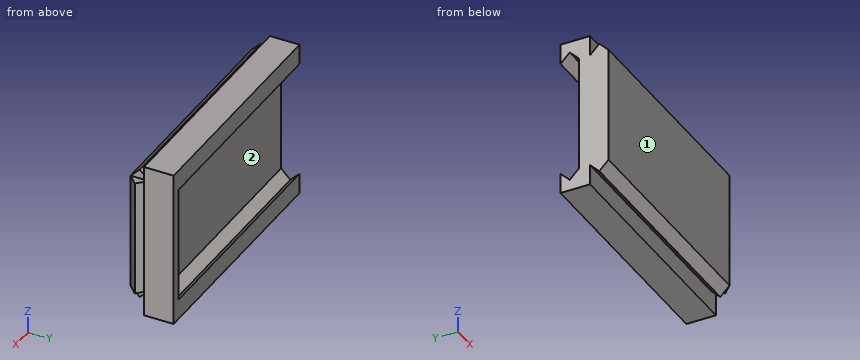
Autodesk Inventor part; units mm, degrees
ref_plane "Work Plane2" through (0, 0, 15.75) normal (0, 0, 1) x (1, 0, 0)
ref_plane "YZ Plane" through (0, 0, 0) normal (1, 0, 0) x (0, 1, 0)
ref_plane "XZ Plane" through (0, 0, 0) normal (0, 1, 0) x (-1, 0, 0)
sketch "Sketch5" plane through (0, 0, 0) normal (0, 0, 1) x (1, 0, 0)
  line L0 (-32, -5) -> (32, -5)
  line L1 (32, -5) -> (32, 5)
  line L2 (32, 5) -> (-32, 5)
  line L3 (-32, 5) -> (-32, -5)
  line L4 (-32, -5) -> (32, 5) construction
  line L5 (32, -5) -> (-32, 5) construction
  point P0 (0, 0)
  dimension "d17" = 64
  dimension "d18" = 10
extrude "Extrusion5" add sketch "Sketch5" along normal mid plane 46.5
ref_plane "Work Plane2" through (0, 0, 15.75) normal (0, 0, 1) x (1, 0, 0)
sketch "Sketch7" plane through (0, 0, 15.75) normal (0, 0, 1) x (1, 0, 0)
  line L0 (32, 5) -> (-32, 5)
  line L1 (-32, 5) -> (-32, -5)
  line L2 (-32, -5) -> (32, -5)
  line L3 (32, -5) -> (32, 5)
  line L4 (32, -5) -> (32, 5)
  line L5 (-32, -5) -> (32, -5)
  line L6 (32, 5) -> (-32, 5)
  line L7 (29.5, 5) -> (29.5, 0)
  line L8 (29.5, 5) -> (32, 2.5)
  line L9 (32, 2.5) -> (29.5, 0)
  point P0 (0, 0)
extrude "Extrusion6" cut sketch "Sketch7" against normal blind 31.5 contours L8 L9 L7
sketch "Sketch8" plane through (-32, -5, 23.25) normal (-1, 0, 0) x (0, 0, 1)
  line L0 (-46.5, 10) -> (0, 10)
  line L1 (-46.5, 10) -> (-41.5, 10)
  line L2 (-41.5, 0) -> (-46.5, 0)
  line L3 (-46.5, 5) -> (-46.5, 10)
  line L4 (0, 10) -> (-5, 10)
  line L5 (-46.5, 0) -> (-46.5, 10)
  line L6 (-41.5, 10) -> (-39, 10)
  line L7 (-39, 10) -> (-41.5, 7.5)
  line L8 (-39, 7.5) -> (-39, 5)
  line L9 (-39, 5) -> (-41.5, 7.5)
  line L10 (-5, 10) -> (-7.5, 10)
  line L11 (-7.5, 10) -> (-5, 7.5)
  line L12 (-7.5, 5) -> (-7.5, 7.5)
  line L13 (-5, 7.5) -> (-7.5, 5)
  line L14 (-7.5, 5) -> (-39, 5)
  line L15 (-39, 10) -> (-39, 7.5)
  line L16 (-7.5, 7.5) -> (-7.5, 10)
  line L17 (-39, 10) -> (-7.5, 10)
  line L18 (-39, 10) -> (-7.5, 10)
  line L19 (-7.5, 5) -> (-39, 5)
  line L20 (-39, 5) -> (-7.5, 5)
  point P0 (-23.25, 5)
extrude "Extrusion8" cut sketch "Sketch8" against normal blind 61.5
sketch "Sketch9" plane through (-32, -5, -23.25) normal (-1, 0, 0) x (0, 0, 1)
  line L0 (0, 10) -> (46.5, 10)
  line L1 (0, 10) -> (2, 10)
  line L2 (2, 10) -> (2, 0)
  line L3 (2, 0) -> (0, 0)
  line L4 (0, 0) -> (0, 10)
  line L5 (46.5, 10) -> (44.5, 10)
  line L6 (44.5, 10) -> (44.5, 0)
  line L7 (44.5, 0) -> (46.5, 0)
  line L8 (46.5, 0) -> (46.5, 10)
  point P0 (23.25, 5)
  dimension "d37" = 2
  dimension "d38" = 2
extrude "Extrusion9" cut sketch "Sketch9" against normal through all
sketch "Sketch10" plane through (-32, 0, -15.75) normal (-1, 0, 0) x (0, 0, 1)
  line L0 (-5.5, -5) -> (-5.5, 5)
  line L1 (37, 5) -> (37, -5)
  line L2 (-5.5, -5) -> (37, -5)
  line L3 (37, -5) -> (37, -8)
  line L4 (37, -8) -> (-5.5, -8)
  line L5 (-5.5, -8) -> (-5.5, -5)
  point P0 (15.75, 0)
  dimension "d70" = 3
sketch "Sketch12" plane through (-32, 0, -15.75) normal (-1, 0, 0) x (0, 0, 1)
  line L0 (37, -3) -> (42, -3)
  line L1 (42, -3) -> (42, 5)
  line L2 (42, 5) -> (37, 5)
  line L3 (37, 5) -> (37, -3)
  point P0 (15.75, 0)
  dimension "d56" = 5
  dimension "d59" = 8
revolve "Revolution1" [suppressed]
sketch "Sketch13" plane through (-32, -3, 21.25) normal (-1, 0, 0) x (0, 0, 1)
  line L0 (5, 8) -> (0, 8)
  line L1 (0, 8) -> (0, 0)
  line L2 (0, 0) -> (5, 0)
  line L3 (5, 0) -> (5, 8)
  line L4 (5, 0) -> (5, 8)
  line L5 (5, 4) -> (4, 4)
  point P0 (-21.25, 3)
  dimension "d58" = 1
feature "Snap Fit2" [suppressed]
mirror "Mirror1" [suppressed]
extrude "Extrusion11" add sketch "Sketch10" against normal blind 64
sketch "Sketch14" plane through (-32, 0, -15.75) normal (-1, 0, 0) x (0, 0, 1)
  line L0 (37, -8) -> (37, 5)
  line L1 (31.5, 5) -> (37, 5)
  line L2 (31.5, 5) -> (34, 2.5)
  line L3 (34, 2.5) -> (31.5, 0)
  line L4 (31.5, 0) -> (0, 0)
  line L5 (0, 0) -> (-2.5, 2.5)
  line L6 (-2.5, 2.5) -> (0, 5)
  line L7 (-5.5, 5) -> (0, 5)
  line L8 (-5.5, 5) -> (-5.5, -8)
  line L9 (-5.5, -8) -> (37, -8)
  line L10 (-5.5, -8) -> (37, -8)
  line L11 (0, -3) -> (-2.5, -5.5)
  line L12 (0, -8) -> (-2.5, -5.5)
  line L13 (0, -8) -> (-5.5, -8)
  line L14 (-5.5, 5) -> (-5.5, -8)
  line L15 (-5.5, 0) -> (-5, 0)
  line L16 (-5.5, -3) -> (-5.5, -8)
  line L17 (31.5, -3) -> (34, -5.5)
  line L18 (31.5, -8) -> (34, -5.5)
  line L19 (31.5, -8) -> (37, -8)
  line L20 (37, -3) -> (37, -8)
  line L21 (0, -3) -> (-5.5, -3)
  line L22 (31.5, -3) -> (37, -3)
  line L23 (37, -8) -> (37, 5)
  point P0 (15.75, 0)
extrude "Extrusion12" cut sketch "Sketch14" against normal blind 61.5 contours L9 L18 L17 L22 L0 | L9 L8 L21 L11 L12
sketch "Sketch15" plane through (32, 5, 21.25) normal (1, 0, 0) x (0, 0, -1)
  line L0 (0, -13) -> (42.5, -13)
  line L1 (0, -13) -> (5.5, -13)
  line L2 (5.5, -13) -> (5.5, -8)
  line L3 (5.5, -8) -> (0, -8)
  line L4 (0, -8) -> (0, -13)
  line L5 (42.5, -13) -> (42.5, -8)
  line L6 (42.5, -13) -> (37, -13)
  line L7 (37, -13) -> (37, -8)
  line L8 (37, -8) -> (42.5, -8)
  line L9 (42.5, -8) -> (42.5, -13)
  point P0 (21.25, -5)
  dimension "d76" = 5.5
  dimension "d77" = 5
  dimension "d78" = 5.5
  dimension "d79" = 5
extrude "Extrusion13" cut sketch "Sketch15" against normal blind 2.5
sketch "Sketch16" plane through (32, -8, 15.75) normal (0, 0, 1) x (1, 0, 0)
  line L0 (-2.5, 5) -> (-2.5, 2.5)
  line L1 (-2.5, 5) -> (0, 2.5)
  line L2 (0, 0) -> (0, 5)
  line L3 (-64, 0) -> (-2.5, 0)
  line L4 (-2.5, 0) -> (0, 2.5)
  line L5 (0, 5) -> (-64, 5)
  line L6 (-2.5, 5) -> (0, 5)
  line L7 (0, 5) -> (0, 0)
  line L8 (0, 0) -> (-2.5, 0)
  point P0 (-32, 8)
extrude "Extrusion14" cut sketch "Sketch16" against normal through all
properties part number "Enclosure-Bottom"
Could you check a few things on this model? Use its own coordinates, in mm. Face numbers are marked on the shaded views. A direction names the side the tool comes from. Coordinates: 2 decimals unless noted, no trailing zeros. Order: outer loops, then holes, each group sorted by start corner. A loop starts at its lowest first (then second) coordinate and runs counter-clockwise, first axis right, second up. Notation, with made-up numbers: (-28.75, 23) -> (-21.75, 23) arc R15 ccw to (-21.75, 44) -> close; hole circle Ø10 at (78.5, 2). An arc over 180 degrees is marked (long way). One line per item, written item: value. Start each with the question number.
1) Imagine slicing it at C-C on x = -11. List the corners of the cut face in (y, z) for me, plus the area to 3 significant figures.
2) Which directions (+Z, -Z, +X, -X, +Y, -Y) give clear straight access to the entire face, cutting with the end or side of a thin tool? Please do the marked faces 1 and 2.
3) Imagine slicing it at B-B on y = 1.75. List the corners of the cut face in (x, z) for me, plus the area to 3 significant figures.
4) I'm going to push flat-ended pins straight in: pin 1 (1.2 mm diameter, centred on x = 30.5, y = -6, fed in from -Z); pin 2 (0.8 mm diameter, centred on x = 30.5, y = -6.5, fed in from +Z); pin 3 (9.5 mm diameter, centred on x = -13, z = -2.5, fed in from +Y). Where does each tip first touch, or does it pass through?
5) Imagine slicing it at D-D on y = -4.5. List the corners of the cut face in (x, z) for me, plus the area to 3 significant figures.
6) If I drill on L1, parallel to Y at x = 24, z = 3.5; L2, parallel to Y at x = -28.5, z = 16; L3, parallel to Z at x = 14, y = 1.25, over which ranges is the centre line in solid material (lowest first)? Write a range as [from, to].
Answer list:
1. outline: (-8, -15.75) -> (-5.5, -18.25) -> (-3, -15.75) -> (-3, -21.25) -> (5, -21.25) -> (5, -15.75) -> (2.5, -18.25) -> (0, -15.75) -> (0, 15.75) -> (2.5, 18.25) -> (5, 15.75) -> (5, 21.25) -> (-3, 21.25) -> (-3, 15.75) -> (-5.5, 18.25) -> (-8, 15.75) -> close
1. area: 340 mm2
2. face 1: +Z, -Z, +X, -X, -Y
2. face 2: -X, +Y
3. outline: (-32, -21.25) -> (32, -21.25) -> (32, 21.25) -> (-32, 21.25) -> (-32, 17.5) -> (29.5, 17.5) -> (29.5, 15.75) -> (31.25, 15.75) -> (31.25, -15.75) -> (29.5, -15.75) -> (29.5, -17.5) -> (-32, -17.5) -> close
3. area: 512 mm2
4. pin 1: stops at z = -15.75
4. pin 2: stops at z = 15.75
4. pin 3: stops at y = 0
5. outline: (-32, -17.25) -> (29.5, -17.25) -> (29.5, -15.75) -> (31, -15.75) -> (31, 15.75) -> (29.5, 15.75) -> (29.5, 17.25) -> (-32, 17.25) -> close
5. area: 2,170 mm2
6. L1: y = [-8, 0]
6. L2: y = [-7.75, -3.25], [-3, 0.25], [4.75, 5]
6. L3: z = [-21.25, -17], [17, 21.25]
